Build history of the part. All positions in model axes, mm. Face numbers are marked on the shaded views. A direction names the side the tool comes from. Give positions to 0.01 mm unless a question says otherwise; leave off trailing zeros. Order: outer loops, then holes, each group sorted by start corner. A loop starts at its lowest first (then second) coordinate and runs counter-clockwise, first axis right, second up. Notation, with made-up numbers: (68, -19.75) - (124, -19.75) arc R9 ccw to (124, -11.75) - close; hole circle Ø1 at (-22.5, 65.5). An arc over 180 degrees is marked (long way). Use a Markdown table: item, result.
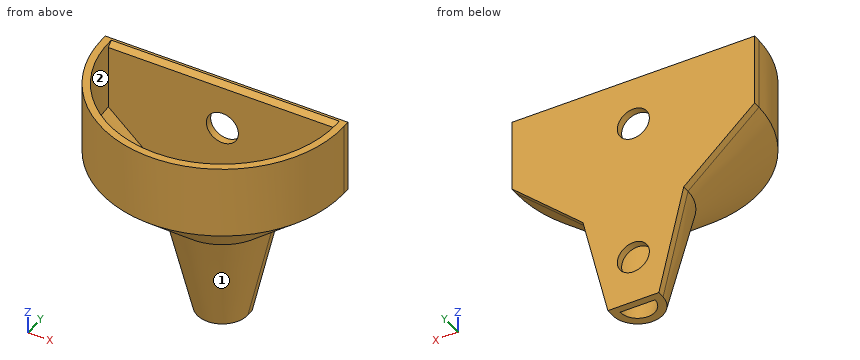
from build123d import *

# Parameters (mm, degrees)
F2_W        = 80.1923088729
F2_H        = 33.5576944053
F3_DEPTH    = 69.4
F5_DEPTH    = 1.5
F6_R        = 3.3
F7_DEPTH    = 3
F8_T4_DEPTH = 52.1433659759
F8_S5_R     = 23.5
F8_T6_DEPTH = 28


# Not quite as in the source:
# - a fillet or chamfer that OpenCascade refuses, or shapes differently, is made with other operations: its cross-section is extruded or revolved along the edge and cut away or added


with BuildPart() as f1:
    # F0 (on Front) → F1 (revolve)
    with BuildSketch(Plane.XZ):
        Polygon((-23.5, 35.6656860253), (-23.5, 48.5), (-23.5, 50), (-25, 50), (-25, 35), (-10.384612577, 21.7765538924), (-5.247530064, 0), (-3.5904949309, 0), (-8.884612577, 22.4422399178), align=None)
    revolve(axis=Axis((0, 0, 32.1634635329), (0, 0, 1)))

    # F2 (on Top) → F3 (cut)
    with BuildSketch(Plane.XY):
        with Locations((8.9423079044, 16.7788472027)):
            Rectangle(F2_W, F2_H)
    extrude(amount=F3_DEPTH, mode=Mode.SUBTRACT)

    # F4 (on face) → F5 (join)
    with BuildSketch(Plane(origin=(0, 0, 0), x_dir=(-1, 0, 0), z_dir=(0, 1, 0))):
        Polygon((25, 50), (-25, 50), (-25, 35), (-10.384612577, 21.7765538924), (-5.247530064, 0), (5.247530064, 0), (10.384612577, 21.7765538924), (25, 35), align=None)
    extrude(amount=F5_DEPTH)

    # F6 (on face) → F7 (cut)
    with BuildSketch(Plane(origin=(0, 1.5, 0), x_dir=(-1, 0, 0), z_dir=(0, 1, 0))):
        with Locations((0, 40)):
            Circle(F6_R)
        with Locations((0, 10)):
            Circle(F6_R)
    extrude(amount=-F7_DEPTH, mode=Mode.SUBTRACT)

    # F8: chamfer of 1 on 1 edges, made by hand


with BuildPart() as f8_tool2:
    # F8_s3 → F8_t4 (new body)
    with BuildSketch(Plane.YZ.offset(-26.071682988)):
        Polygon((0, 49), (1, 50), (0, 50), align=None)
    extrude(amount=F8_T4_DEPTH)

    # F8_s5 → F8_t6 (intersect, symmetric)
    with BuildSketch(Plane.XY.offset(49.5)):
        Circle(F8_S5_R)
    extrude(amount=F8_T6_DEPTH, both=True, mode=Mode.INTERSECT)


with BuildPart() as f1_1:
    add(f1.part)

    # F8_t1: cut F8_tool2
    add(f8_tool2.part, mode=Mode.SUBTRACT)


solid = f1_1.part
1) Pin check, flat tips, straight feed: P1, Ø10.5, axis at x = 0, z = 10, coming from the -Y side (3 decimals); P2, Ø3, axis at y = -2, z = 22, coming from the +X side; P3, Ø1, axis at x = 3.5, z = 36, coming from the -Y side. Stop position of each tip, or through.
Computed:
| item | result |
|---|---|
| P1 | stops at y = -8.845 |
| P2 | stops at x = 12.14 |
| P3 | stops at y = -24.82 |
2) Wall check: line 1 (Z direction, x = 0, y = 0.6); line 2 (Z direction, x = 0, y = 0.9); line 3 (X direction, y = -1, z = 36.5). Give the ranges that are in metal, low to high. Write a range as from..to.
Computed:
| item | result |
|---|---|
| line 1 | z = 0..6.7, 13.3..36.7, 43.3..49.6 |
| line 2 | z = 0..6.7, 13.3..36.7, 43.3..49.9 |
| line 3 | x = -24.98..-23.48, 23.48..24.98 |
3) Slice it at A-A (z = 40). Write the cut outline in (x, y), and give its area (3 significant figures).
Computed:
| item | result |
|---|---|
| outline | (-25, 0) arc R25 ccw to (25, 0) - (25, 1.5) - (3.3, 1.5) - (3.3, 0) - (23.5, 0) arc R23.5 cw to (-23.5, 0) - (-3.3, 0) - (-3.3, 1.5) - (-25, 1.5) - close |
| area | 179 mm² |
4) Tool access for the marked faces 1 and 2: list every direction of +Z, -Z, +X, -X, +Y, -Y with a clear straight run to the whole face (end or side of a thin tool).
Computed:
| item | result |
|---|---|
| face 1 | -Z, -Y |
| face 2 | +Z |
5) Slice it at C-C (z = 23.5). Write the cut outline in (x, y).
Computed:
| item | result |
|---|---|
| outline | (-12.29, 0) arc R12.29 ccw to (12.29, 0) - (12.29, 1.5) - (-12.29, 1.5) - close; hole (-10.05, 0) arc R10.05 ccw to (10.05, 0) - close |
6) Slice it at B-B (x = 0). Write the cut outline in (y, z).
Computed:
| item | result |
|---|---|
| outline | (-25, 35) - (-10.38, 21.78) - (-5.25, 0) - (-3.59, 0) - (-8.88, 22.44) - (-23.5, 35.67) - (-23.5, 50) - (-25, 50) - close; (0, 0) - (1.5, 0) - (1.5, 6.7) - (0, 6.7) - close; (0, 13.3) - (1.5, 13.3) - (1.5, 36.7) - (0, 36.7) - close; (0, 43.3) - (1.5, 43.3) - (1.5, 50) - (1, 50) - (0, 49) - close |
7) Slice it at D-D (z = 33.5). Write the cut outline in (x, y), and give its area (3 significant figures).
Computed:
| item | result |
|---|---|
| outline | (-23.34, 0) arc R23.34 ccw to (23.34, 0) - (23.34, 1.5) - (-23.34, 1.5) - close; hole (-21.11, 0) arc R21.11 ccw to (21.11, 0) - close |
| area | 226 mm² |
